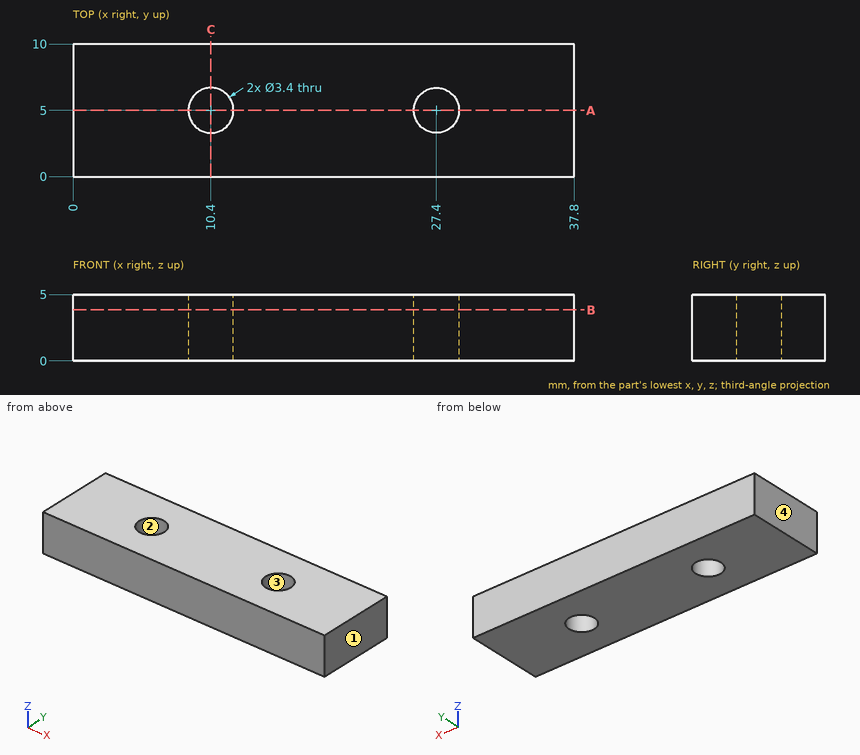
Answer from the drawing. Dimensions are ordinates in mm from the lowest x, y and z of the part. Give positions to 0.01 mm unless a question says otherwise; leave off trailing zeros. Write each loop counter-clockwise with the first axis right and the second up, starting at its lowest first coordinate (ties: lowest second). Pieces come first, ordered by that corner, then holes. Notation, with made-up numbers: (41.25, 45.5) -> (88.25, 45.5) arc R26 cw to (88.25, 80.5) -> close; hole circle Ø4 at (82, 72.25). An arc over 180 degrees is marked (long way). One line per question, with ' | ' between items. Start each with the question number.
1. For a pull along X with two mould halves and no side action, classify the marked faces 1, 2, 3 and 4 as pulls with the +X half, pulls with the -X half, needs draft (parallel to the pull), parting line crosses it, or undercut.
2. Find the intervals of material crossed by probe 1 along Y at (x, z) = (27.4, 2.1); probe 2 along X at (y, z) = (6.5, 2.1); probe 3 along X at (y, z) = (6.25, 0.45), in increasing order.
3. Section B-B (z = 3.85) is taken. Determine the outline of the cut face in (x, y), plus the area to 3 significant figures.
4. Section C-C (x = 10.4) is taken. Determine the outline of the cut face in (y, z), plus the area to 3 significant figures.
5. Section A-A (y = 5) is taken. Determine the outline of the cut face in (x, z).
Response values:
1) face 1: pulls with the +X half | face 2: undercut | face 3: undercut | face 4: pulls with the -X half
2) probe 1: 0 to 3.3, 6.7 to 10 | probe 2: 0 to 9.6, 11.2 to 26.6, 28.2 to 37.8 | probe 3: 0 to 9.25, 11.55 to 26.25, 28.55 to 37.8
3) outline: (0, 0) -> (37.8, 0) -> (37.8, 10) -> (0, 10) -> close; hole circle Ø3.4 at (10.4, 5); hole circle Ø3.4 at (27.4, 5) | area: 360 mm2
4) outline: (0, 0) -> (3.3, 0) -> (3.3, 5) -> (0, 5) -> close; (6.7, 0) -> (10, 0) -> (10, 5) -> (6.7, 5) -> close | area: 33.0 mm2
5) outline: (0, 0) -> (8.7, 0) -> (8.7, 5) -> (0, 5) -> close; (12.1, 0) -> (25.7, 0) -> (25.7, 5) -> (12.1, 5) -> close; (29.1, 0) -> (37.8, 0) -> (37.8, 5) -> (29.1, 5) -> close
